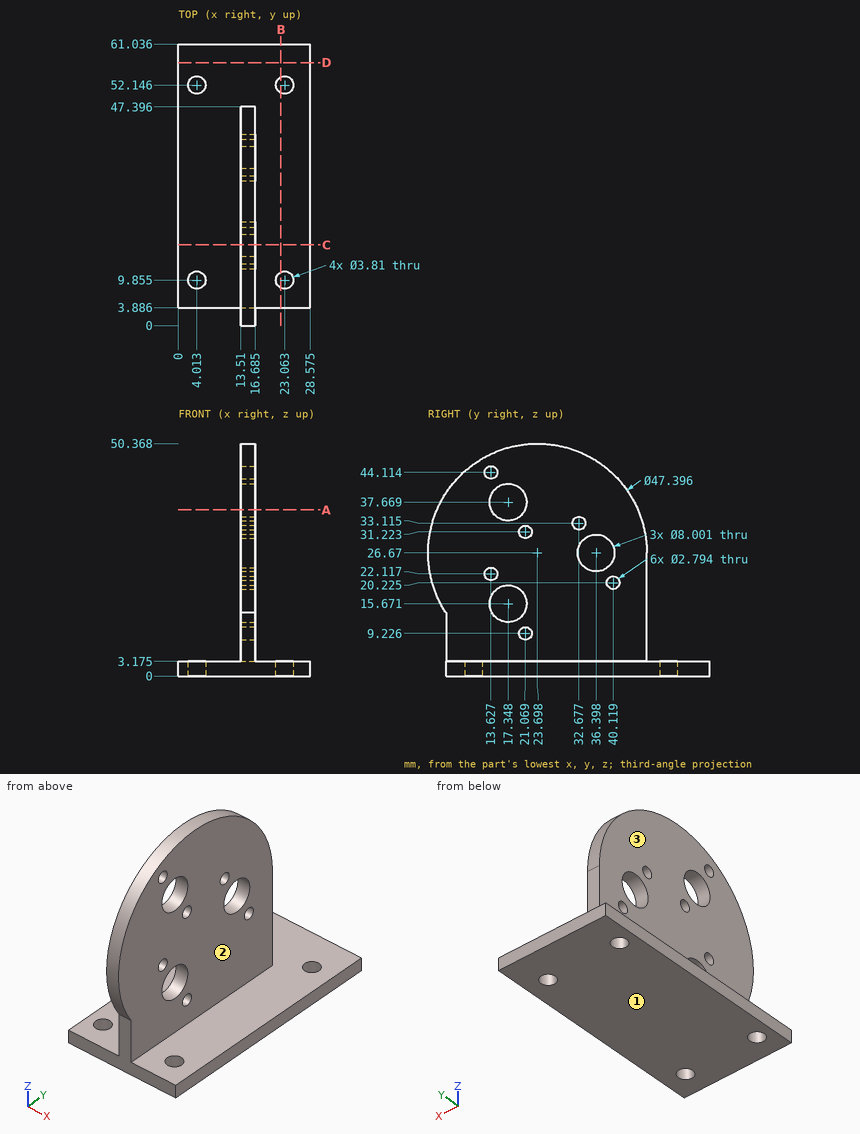
Could you check a few things on this drawing? It's one solid part, dimensions in mm from its lowest x, y, z. A direction names the side the tool comes from. Give positions to 0.01 mm unless a question says otherwise; leave off trailing zeros. Write each loop counter-clockwise with the first axis right and the second up, starting at its lowest first coordinate (ties: lowest second). Pieces come first, ordered by that corner, then holes. Notation, with made-up numbers: (55.25, -29.5) -> (97.25, -29.5) arc R9 cw to (97.25, -18.5) -> close; hole circle Ø6 at (-24.75, 75). An arc over 180 degrees is marked (long way). Answer as CSV lines item,"result". Start each with the question number.
(1) Which directions (+Z, -Z, +X, -X, +Y, -Y) give clear straight access to the entire face, cutting with the end or side of a thin tool? Please do the marked faces 1, 2 and 3.
(2) Please list where these lines run through material, in increasing order: line 1 (Z direction, x = 26.25, y = 42) (1 decimal); line 2 (X direction, y = 37, z = 45) (1 decimal); line 3 (Y direction, x = 13.75, z = 11).
(3) I'm going to push flat-ended pins straight in: pin 1 Ø6 at (y, z) = (46.5, 39) entering from +X (3 decimals); pin 2 Ø3.5 at (y, z) = (40.12, 20.22) entering from -X; pin 3 Ø2.5 at (y, z) = (21.07, 9.23) entering from -X; pin 4 Ø10 at (x, z) = (10.5, 28) entering from +Y. Where does each tip first touch, or does it pass through?
(4) If we section it at B-B, the plane x = 22.25: Write out the boundary of the cut face in (y, z) (1 decimal).
(5) If we section it at D-D, the plane y = 57: Write out the boundary of the cut face in (x, z) (1 decimal).
(6) If we section it at A-A, the plane z = 36: Write out the boundary of the cut face in (x, y) (1 decimal).
(7) If we section it at C-C, the plane y = 17.5: Write out the boundary of the cut face in (x, z) (1 decimal), and give its area (3 significant figures).
Answer list:
1,face 1,"-Z, +X, -X, +Y, -Y"
1,face 2,"+Z, +X, +Y, -Y"
1,face 3,"+Z, -X, +Y, -Y"
2,line 1,"0 to 3.2"
2,line 2,"13.5 to 16.7"
2,line 3,"3.89 to 47.4"
3,pin 1,"x = 16.685"
3,pin 2,"x = 13.51"
3,pin 3,"through"
3,pin 4,"y = 47.4"
4,outline,"(3.9, 0) -> (8.1, 0) -> (8.1, 3.2) -> (3.9, 3.2) -> close; (11.6, 0) -> (50.4, 0) -> (50.4, 3.2) -> (11.6, 3.2) -> close; (53.9, 0) -> (61, 0) -> (61, 3.2) -> (53.9, 3.2) -> close"
5,outline,"(0, 0) -> (28.6, 0) -> (28.6, 3.2) -> (0, 3.2) -> close"
6,outline,"(13.5, 1.9) -> (16.7, 1.9) -> (16.7, 13.7) -> (13.5, 13.7) -> close; (13.5, 21) -> (16.7, 21) -> (16.7, 45.5) -> (13.5, 45.5) -> close"
7,outline,"(0, 0) -> (28.6, 0) -> (28.6, 3.2) -> (16.7, 3.2) -> (16.7, 11.7) -> (13.5, 11.7) -> (13.5, 3.2) -> (0, 3.2) -> close; (13.5, 19.7) -> (16.7, 19.7) -> (16.7, 33.7) -> (13.5, 33.7) -> close; (13.5, 41.7) -> (16.7, 41.7) -> (16.7, 49.5) -> (13.5, 49.5) -> close"
7,area,"187 mm^2"
